from build123d import *

# Parameters (mm, degrees)
BOSS_EXTRUDE1_DEPTH = 5
SKETCH3_R           = 2
CUT_EXTRUDE1_DEPTH  = 5
SKETCH4_R           = 1
CUT_EXTRUDE9_DEPTH  = 61


with BuildPart() as part:
    # Sketch1 → Boss-Extrude1 (new body)
    with BuildSketch(Plane.XY):
        Polygon((53, -5), (54, -5), (54.932615316, -7), (56.067384684, -7), (57, -5), (60, -5), (60, 0), (57, 0), (56.067384684, 2), (54.932615316, 2), (54, 0), (53, 0), (52.067384684, 2), (50.932615316, 2), (50, 0), (49, 0), (48.067384684, 2), (46.932615316, 2), (46, 0), (45, 0), (44.067384684, 2), (42.932615316, 2), (42, 0), (41, 0), (40.067384684, 2), (38.932615316, 2), (38, 0), (37, 0), (36.067384684, 2), (34.932615316, 2), (34, 0), (33, 0), (32.067384684, 2), (30.932615316, 2), (30, 0), (20, 0), (20, -5), (30, -5), (30.932615316, -7), (32.067384684, -7), (33, -5), (34, -5), (34.932615316, -7), (36.067384684, -7), (37, -5), (38, -5), (38.932615316, -7), (40.067384684, -7), (41, -5), (42, -5), (42.932615316, -7), (44.067384684, -7), (45, -5), (46, -5), (46.932615316, -7), (48.067384684, -7), (49, -5), (50, -5), (50.932615316, -7), (52.067384684, -7), align=None)
    extrude(amount=BOSS_EXTRUDE1_DEPTH)

    # Sketch3 → Cut-Extrude1 (cut)
    with BuildSketch(Plane(origin=(60, 0, 0), x_dir=(0, 0, -1), z_dir=(1, 0, 0))):
        with Locations((-2.601693616, -2.5)):
            Circle(SKETCH3_R)
    extrude(amount=-CUT_EXTRUDE1_DEPTH, mode=Mode.SUBTRACT)

    # Sketch4 → Cut-Extrude9 (cut, through all)
    with BuildSketch(Plane(origin=(0, 0, 0), x_dir=(0, 0, -1), z_dir=(1, 0, 0))):
        with Locations((-2.601693616, -2.5)):
            Circle(SKETCH4_R)
    extrude(amount=CUT_EXTRUDE9_DEPTH, mode=Mode.SUBTRACT)


solid = part.part
Source: CAD feature listing. Evaluate the final solid. Frame: model axes, mm. A direction names the side the tool comes from. Round coordinates to 2 decimals unless told otherwise and drop trailing zeros. Write each loop counter-clockwise with the first axis right and the second up, starting at its lowest first coordinate (ties: lowest second). Pieces come first, ordered by that corner, then holes. Notation, with made-up numbers: (79.25, -34.75) - (121.25, -34.75) arc R18 ccw to (121.25, -6.75) - close; hole circle Ø7 at (56, -27.5). An arc over 180 degrees is marked (long way). Use CSV: the item, a comma, the result in double quotes. Start each with the question number.
(1) Material intervals for probe 1 along Z at (x, y) = (28, -2.5); probe 2 along X at (y, z) = (-2.75, 4.5); probe 3 along Y at (x, z) = (24.5, 2.6), sorted ascending. Write a range as [from, to].
(2) Cut plane A-A, the plane y = -2.5. Return loops of the section in (x, z), and give its area (3 significant figures).
(3) First-contact query: pin 1 Ø2.5 at (x, z) = (58.5, 3.5) entering from +Y; pin 2 Ø1.1 at (x, z) = (41.5, 3) entering from +Y; pin 3 Ø1.1 at (x, z) = (49.5, 2) entering from -Y. Flat tips, straight axial feed; report the tip coordinate or a pass-through.
(4) Mould query, pull axis X, two halves, no side actions, for faces 4 (the face through (30.46, -5.99, 2.46)), 5 (the face through (41.5, 0, 2.5)), 6 (the face through (25, 0, 2)). Classes: pulls with the +X half, pulls with the -X half, needs draft (parallel to the pull), parting line crosses it, or undercut.
(5) Set-up query: faces 1 (the face through (25, -5, 2)), 2 (the face through (48.53, -6.01, 2.46)), 3 (the face through (57.5, -3.7, 4.2)). Return all of +Z, -Z, +X, -X, +Y, -Y with unobstructed straight access to the full face (end or side cutting, diameter ignored); none if empty.
(6) Cut plane D-D, the plane y = 0.75. Return loops of the section in (x, z), and give its area (3 significant figures).
(7) Cut plane C-C, the plane x = 26. Return loops of the section in (y, z).
(8) Cut plane B-B, the plane y = -6. Return loops of the section in (x, z).
Geometry says:
1,probe 1,"[0, 1.6], [3.6, 5]"
1,probe 2,"[20, 55]"
1,probe 3,"[-5, -3.5], [-1.5, 0]"
2,outline,"(20, 0) - (60, 0) - (60, 0.6) - (55, 0.6) - (55, 1.6) - (20, 1.6) - close; (20, 3.6) - (55, 3.6) - (55, 4.6) - (60, 4.6) - (60, 5) - (20, 5) - close"
2,area,"110 mm²"
3,pin 1,"y = 0"
3,pin 2,"y = 0.11"
3,pin 3,"y = -5.11"
4,face 4,"pulls with the -X half"
4,face 5,"undercut"
4,face 6,"needs draft"
5,face 1,"+Z, -Z, -X, -Y"
5,face 2,"+Z, -Z, -Y"
5,face 3,"+X"
6,outline,"(30.35, 0) - (32.65, 0) - (32.65, 5) - (30.35, 5) - close; (34.35, 0) - (36.65, 0) - (36.65, 5) - (34.35, 5) - close; (38.35, 0) - (40.65, 0) - (40.65, 5) - (38.35, 5) - close; (42.35, 0) - (44.65, 0) - (44.65, 5) - (42.35, 5) - close; (46.35, 0) - (48.65, 0) - (48.65, 5) - (46.35, 5) - close; (50.35, 0) - (52.65, 0) - (52.65, 5) - (50.35, 5) - close; (54.35, 0) - (56.65, 0) - (56.65, 5) - (54.35, 5) - close"
6,area,"80.5 mm²"
7,outline,"(-5, 0) - (0, 0) - (0, 5) - (-5, 5) - close; hole circle Ø2 at (-2.5, 2.6)"
8,outline,"(30.47, 0) - (32.53, 0) - (32.53, 5) - (30.47, 5) - close; (34.47, 0) - (36.53, 0) - (36.53, 5) - (34.47, 5) - close; (38.47, 0) - (40.53, 0) - (40.53, 5) - (38.47, 5) - close; (42.47, 0) - (44.53, 0) - (44.53, 5) - (42.47, 5) - close; (46.47, 0) - (48.53, 0) - (48.53, 5) - (46.47, 5) - close; (50.47, 0) - (52.53, 0) - (52.53, 5) - (50.47, 5) - close; (54.47, 0) - (56.53, 0) - (56.53, 5) - (54.47, 5) - close"
